Input: part model. Units: mm. Frame: model coordinates. A direction names the side the tool comes from. Round coordinates to 2 decimals unless told otherwise and drop trailing zeros. Order: outer loops, then holes, each group sorted by start corner. A loop starts at its lowest first (then second) coordinate and runs counter-clockwise, first axis right, second up.
Item 1: Cut plane B-B on y = -16.5. Output: boundary loops of the cut face in (x, z), then the cut area to 3 significant figures.
Item 2: Reachability of faces 1 (the flat face through (-33, 0, 2)), 2 (the flat face through (107, 0, -2.9)), 3 (the flat face through (0.666, 0, 6)), 4 (the flat face through (-6, 9.9, 7)), 5 (the flat face through (-6, -9.9, 7)) from +Z, -Z, +X, -X, +Y, -Y: full face, straight path, thin tool, end or side. Return the list, or none.
Item 3: Mould query, pull axis X, two halves, no side actions, for faces 6 (the flat face through (49, -13, 4)), 7 (the flat face through (-53.338, 0, 6)), 8 (the cylindrical face through (29.1, -12.64, 2.03)), 9 (the cylindrical face through (102.666, 0.176, -3.895)). Classes: released by +X, released by -X, zero draft, split by the parting line, or undercut.
Item 4: Cut plane A-A on x = 83.5. Output: boundary loops of the cut face in (y, z), then the cut area to 3 significant figures.
Item 5: First-contact query: pin 1 (2 mm diameter, centred on x = -22.5, y = -3.5, fed in from +Z); pin 2 (1.5 mm diameter, centred on x = -29.5, y = -15, fed in from +Z); pin 3 (10 mm diameter, centred on y = 11, z = -2, fed in from -X); pin 4 (4 mm diameter, centred on y = -1, z = 0.5, fed in from -X). Flat tips, straight axial feed; report the tip coordinate or a pass-through.
Item 6: Cut plane C-C on x = -15.5. Output: boundary loops of the cut face in (y, z), then the cut area to 3 significant figures.
Item 7: Cut plane D-D on y = 0. Give the number of separate pieces and of enclosed holes in the cut face, then the cut area to 3 significant figures.
Item 8: Line query: L1, parallel to X at y = 0, z = 1.5; L2, parallel to Z at x = -37.5, y = -15.5; L3, parallel to Z at x = -32, y = -9.5. Output: solid intervals per line, ascending.
Autodesk Inventor part; units mm, degrees
ref_plane "YZ Plane" through (0, 0, 0) normal (1, 0, 0) x (0, 1, 0)
ref_plane "XZ Plane" through (0, 0, 0) normal (0, 1, 0) x (-1, 0, 0)
ref_plane "XY Plane" through (0, 0, 0) normal (0, 0, 1) x (1, 0, 0)
sketch "Sketch1" plane through (0, 0, 0) normal (0, 0, 1) x (1, 0, 0)
  line L0 (-43.3376, 0) -> (106.6624, 0) construction
  line L1 (-43.3376, -20) -> (106.6624, -20)
  line L2 (106.6624, 20) -> (-43.3376, 20)
  arc A0 (-43.3376, 20) -> (-43.3376, -20) centre (-43.3376, 0) ccw
  arc A1 (106.6624, -20) -> (106.6624, 20) centre (106.6624, 0) ccw
  point P0 (0, 0)
  point P1 (31.6624, 0)
  dimension "d0" = 150
  dimension "d1" = 20
extrude "Extrusion1" add sketch "Sketch1" along normal blind 4
sketch "Sketch2" plane through (0, 0, 4) normal (0, 0, 1) x (1, 0, 0)
  arc A0 (-43.3376, 20) -> (-43.3376, -20) centre (-43.3376, 0) ccw
  arc A1 (106.6624, -20) -> (106.6624, 20) centre (106.6624, 0) ccw
  circle A2 centre (-43.3376, 0) radius 6.4
  circle A3 centre (106.6624, 0) radius 4
  point P0 (0, 0)
  dimension "d4" = 12.8
  dimension "d5" = 8
extrude "Extrusion2" add sketch "Sketch2" against normal blind 11.9 contours A3
sketch "Sketch5" plane through (0, 0, 4) normal (0, 0, 1) x (1, 0, 0)
  line L0 (-43.3376, -20) -> (106.6624, -20)
  arc A0 (92.1536, -20) -> (-35.7554, -20) centre (28.1991, -294.1981) ccw
  point P0 (0, 0)
extrude "Extrusion5" cut sketch "Sketch5" against normal through all
sketch "Sketch6" plane through (0, 0, 0) normal (0, 0, -1) x (-1, 0, 0)
  point P0 (0, 0)
sketch "Sketch7" plane through (106.6624, 0, -7.9) normal (0, 0, -1) x (-1, 0, 0)
  circle A0 centre (0, 0) radius 2.7
  point P0 (106.6624, 0)
  dimension "d18" = 5.4
extrude "Extrusion6" cut sketch "Sketch7" against normal blind 5
sketch "Sketch8" plane through (0, 0, 0) normal (0, 0, -1) x (-1, 0, 0)
  point P0 (0, 0)
extrude "Extrusion7" cut sketch "Sketch2" along normal mid plane 11.9 contours A2
sketch "Sketch9" plane through (106.6624, 0, -7.9) normal (0, 0, -1) x (-1, 0, 0)
  point P0 (106.6624, 0)
sketch "Sketch10" plane through (0, 0, 0) normal (0, 0, -1) x (-1, 0, 0)
  point P0 (0, 0)
sketch "Sketch11" plane through (0, 0, 4) normal (0, 0, 1) x (1, 0, 0)
  line L0 (-70.0866, 9.9) -> (0.6664, 9.9)
  line L1 (0.6664, 9.9) -> (0.6664, -9.9)
  line L2 (0.6664, -9.9) -> (-70.0866, -9.9)
  line L3 (-70.0866, -9.9) -> (-70.0866, 9.9)
  line L4 (-70.0866, 9.9) -> (0.6664, -9.9) construction
  line L5 (0.6664, 9.9) -> (-70.0866, -9.9) construction
  circle A0 centre (-43.3376, 0) radius 6.4
  point P0 (0, 0)
  point P1 (-34.7101, 0)
  dimension "d23" = 70.753
  dimension "d24" = 19.8
  dimension "d25" = 26.749
  dimension "d26" = 9.9
sketch "Sketch12" plane through (0, 0, 4) normal (0, 0, 1) x (1, 0, 0)
  circle A0 centre (-43.3376, 0) radius 6.4
  point P0 (0, 0)
ref_plane "Work Plane1" through (0, 0, 2) normal (0, 0, 1) x (1, 0, 0)
sketch "Sketch13" plane through (0, 0, 2) normal (0, 0, 1) x (1, 0, 0)
  arc A0 (-43.3376, 20) -> (-60.7155, 9.9) centre (-43.3376, 0) ccw
  line L0 (-43.3376, 20) -> (-59.4218, 20)
  line L1 (-59.4166, -20.0032) -> (-43.3376, -20.0032)
  line L2 (-43.3376, -20.0032) -> (-43.3376, 20)
  circle A1 centre (-43.3376, 0) radius 4
  arc A2 (-59.4218, 20) -> (-59.4166, -20.0032) centre (-47.3376, 0) ccw
  point P0 (0, 0)
  point P1 (-43.3376, -4)
  point P2 (-43.3376, 4)
extrude "Extrusion9" add sketch "Sketch13" along normal mid plane 4 contours L2 A1 L1 A2 L0
extrude "Extrusion10" cut sketch "Sketch11" against normal blind 2
sketch "Sketch14" plane through (0, 0, 2) normal (0, 0, 1) x (1, 0, 0)
  line L0 (-53.3376, 9.9) -> (-70.0866, 9.9)
  line L1 (-70.0866, 9.9) -> (-70.0866, -9.9)
  line L2 (-70.0866, -9.9) -> (-53.3376, -9.9)
  line L3 (-53.3376, -9.9) -> (-53.3376, 9.9)
  line L4 (-53.3376, 9.9) -> (-70.0866, -9.9) construction
  line L5 (-70.0866, 9.9) -> (-53.3376, -9.9) construction
  arc A0 (-43.3376, -6.4) -> (-43.3376, 6.4) centre (-43.3376, 0) ccw
  line L6 (-12.7376, 9.9) -> (0.6624, 9.9)
  line L7 (0.6624, 9.9) -> (0.6624, -9.9)
  line L8 (0.6624, -9.9) -> (-12.7376, -9.9)
  line L9 (-12.7376, -9.9) -> (-12.7376, 9.9)
  line L10 (-12.7376, 9.9) -> (0.6624, -9.9) construction
  line L11 (0.6624, 9.9) -> (-12.7376, -9.9) construction
  point P0 (0, 0)
  point P1 (-61.7121, 0)
  point P2 (-61.7121, -9.9)
  point P3 (-6.0376, 0)
  dimension "d33" = 19.8
  dimension "d34" = 16.749
  dimension "d35" = 10
  dimension "d36" = 13.4
  dimension "d37" = 19.8
  dimension "d38" = 30.6
extrude "Extrusion11" add sketch "Sketch14" along normal blind 7.5
fillet "Fillet3" radius 14.75 1 edges at (-70.0866, 0, 9.5)
sketch "Sketch15" plane through (0, 0, 2) normal (0, 0, 1) x (1, 0, 0)
  line L0 (0.6664, -9.9) -> (0.6624, -9.9)
  line L1 (0.6664, 9.9) -> (0.6664, -9.9)
  line L2 (0.6624, -9.9) -> (0.6664, -9.9)
  line L3 (0.6664, -9.9) -> (0.6664, 9.9)
  line L4 (0.6664, 9.9) -> (0.6624, 9.9)
  line L5 (0.6624, 9.9) -> (0.6624, -9.9)
  point P0 (0, 0)
extrude "Extrusion12" add sketch "Sketch15" along normal blind 5.5
sketch "Sketch16" plane through (0, 0, 9.5) normal (0, 0, 1) x (1, 0, 0)
  circle A0 centre (-57.9276, -5) radius 1.475
  circle A1 centre (-57.9276, 5) radius 1.475
  line L0 (-58.5975, -9.9) -> (-58.5975, 9.9)
  line L1 (-58.5975, -9.9) -> (-53.3376, -9.9)
  line L2 (-53.3376, 9.9) -> (-58.5975, 9.9)
  circle A2 centre (-8.1476, -5) radius 1.475
  circle A3 centre (-8.1476, 5) radius 1.475
  line L3 (-12.7376, 9.9) -> (-12.7376, -9.9)
  line L4 (-12.7376, -9.9) -> (0.6664, -9.9)
  line L5 (0.6664, 9.9) -> (-12.7376, 9.9)
  arc A4 (-43.3376, -6.4) -> (-43.3376, 6.4) centre (-43.3376, 0) ccw
  point P0 (0, 0)
  dimension "d44" = 2.95
  dimension "d45" = 2.95
  dimension "d47" = 4.9
  dimension "d49" = 4.9
  dimension "d50" = 2.95
  dimension "d51" = 2.95
  dimension "d52" = 4.59
  dimension "d53" = 4.59
  dimension "d54" = 4.9
  dimension "d55" = 4.9
  dimension "d60" = 14.59
  dimension "d61" = 14.59
extrude "Extrusion13" cut sketch "Sketch16" against normal blind 10
sketch "Sketch17" plane through (0, 0, 2) normal (0, 0, 1) x (1, 0, 0)
  point P0 (0, 0)
sketch "Sketch18" plane through (0, 0, 2) normal (0, 0, 1) x (1, 0, 0)
  point P0 (0, 0)
extrude "Extrusion14" cut sketch "Sketch12" against normal blind 11.9
sketch "Sketch19" plane through (0, 0, 4) normal (0, 0, 1) x (1, 0, 0)
  circle A0 centre (20.9836, 3.8774) radius 12.933
  circle A1 centre (50.1781, 3.8774) radius 12.933
  circle A2 centre (77.9924, 3.8774) radius 10.5714
  point P0 (0, 0)
extrude "Extrusion15" cut sketch "Sketch19" against normal blind 10
sketch "Sketch20" plane through (0, 0, 2) normal (0, 0, 1) x (1, 0, 0)
  point P0 (0, 0)
properties part number "elbow" material "Aluminum 6061"
From the geometry:
1. outline: (-63.88, 0) - (-18.26, 0) - (-18.26, 4) - (-63.88, 4) - close; (74.66, 0) - (117.97, 0) - (117.97, 4) - (74.66, 4) - close
1. area: 356 mm2
2. face 1: +Z
2. face 2: -Z
2. face 3: +Z, +X, +Y, -Y
2. face 4: +Z, +X, -X, +Y
2. face 5: +Z, +X, -X, -Y
3. face 6: zero draft
3. face 7: undercut
3. face 8: undercut
3. face 9: split by the parting line
4. outline: (-18.12, 0) - (-5.15, 0) - (-5.15, 4) - (-18.12, 4) - close; (12.9, 0) - (20, 0) - (20, 4) - (12.9, 4) - close
4. area: 80.3 mm2
5. pin 1: stops at z = 2
5. pin 2: stops at z = 4
5. pin 3: stops at x = -70.09
5. pin 4: stops at x = -70.7
6. outline: (-16.05, 0) - (20, 0) - (20, 4) - (9.9, 4) - (9.9, 2) - (-9.9, 2) - (-9.9, 4) - (-16.05, 4) - close
6. area: 105 mm2
7. separate pieces: 5
7. enclosed holes: 0
7. area: 589 mm2
8. L1: x = -70.7 to -49.74, -36.94 to 8.65, 33.32 to 37.84, 62.52 to 68.16, 87.83 to 126.66
8. L2: z = 0 to 4
8. L3: z = 0 to 2
